Could you check a few things on this model? Use its own coordinates, in mm. Round coordinates to 2 decimals unless told otherwise and drop trailing zeros. Write each loop counter-clockwise with the first axis right and the second up, starting at its lowest first coordinate (ties: lowest second). Pieces come first, ordered by that corner, then holes. Notation, with made-up numbers: (-10.75, 52.25) -> (21.25, 52.25) arc R10 ccw to (21.25, 60.25) -> close; hole circle Ø4 at (69.25, -27). An arc over 180 degrees is marked (long way). Answer in a Markdown table with one row per item. Add a question column.
```python
from build123d import *

# Parameters (mm, degrees)
SKETCH1_R           = 1.5
BOSS_EXTRUDE1_DEPTH = 3
SKETCH4_R           = 1.5
CUT_EXTRUDE4_DEPTH  = 165.076201809


with BuildPart() as part:
    # Sketch1 → Boss-Extrude1 (new body)
    with BuildSketch(Plane(origin=(0, 0, 0), x_dir=(1, 0, 0), z_dir=(0, 1, 0))):
        with BuildLine():
            Line((0, 4), (160, 4))
            ThreePointArc((160, 4), (164, 0), (160, -4))
            Line((160, -4), (0, -4))
            ThreePointArc((0, -4), (-4, 0), (0, 4))
        make_face()
        with Locations(Location((0, 0, 0), (0, 0, 270))):
            Circle(SKETCH1_R, mode=Mode.SUBTRACT)
        with Locations(Location((160, 0, 0), (0, 0, 270))):
            Circle(SKETCH1_R, mode=Mode.SUBTRACT)
        with Locations(Location((120, 0, 0), (0, 0, 270))):
            Circle(SKETCH1_R, mode=Mode.SUBTRACT)
    extrude(amount=BOSS_EXTRUDE1_DEPTH)

    # Sketch4 → Cut-Extrude4 (cut, through all)
    with BuildSketch(Plane(origin=(0, 0, 0), x_dir=(1, 0, 0), z_dir=(0, 1, 0))):
        with Locations(Location((40, 0, 0), (0, 0, 270))):
            Circle(SKETCH4_R)
    extrude(amount=CUT_EXTRUDE4_DEPTH, mode=Mode.SUBTRACT)


solid = part.part
```
(1) I need wall thicknesses on L1, parallel to X at y = 0.65, z = 0; L2, parallel to X at y = 2.3, z = -1.25; L3, parallel to Z at x = 120, y = 2. Which ranges of each line are inside material? Lowest first, please.
(2) Suppose I cut it at A-A, the plane z = 0. Please give me the cut outline in (x, y).
(3) For P1, Ø1, axis at y = 1.5, z = -2.5, coming from the +X side; P2, Ø1.8, axis at x = 160, z = 0, coming from the +Y side, each with a flat end and sliding along its axis, tell me the tip position at first contact or that it passes through.
(4) Suppose I cut it at C-C, the plane y = 1.05. Please give me the cut outline in (x, z).
(5) If we mould it in two halves opening along Z, with no side actions, what happens to faces 1 (the face through (81, 1, 4)), 2 (the face through (164, 1, 0)), 3 (the face through (79, 1, -4)), 4 (the face through (161.487, 1.479, -0.195))? For each: pulls with the +Z half, pulls with the -Z half, needs draft (parallel to the pull), parting line crosses it, or undercut.
(6) Suppose I cut it at B-B, the plane x = 120. Please give me the cut outline in (y, z).
Response:
| question | item | result |
|---|---|---|
| 1 | L1 | -4 to -1.5, 1.5 to 38.5, 41.5 to 118.5, 121.5 to 158.5, 161.5 to 164 |
| 1 | L2 | -3.8 to -0.83, 0.83 to 39.17, 40.83 to 119.17, 120.83 to 159.17, 160.83 to 163.8 |
| 1 | L3 | -4 to -1.5, 1.5 to 4 |
| 2 | outline | (-4, 0) -> (-1.5, 0) -> (-1.5, 3) -> (-4, 3) -> close; (1.5, 0) -> (38.5, 0) -> (38.5, 3) -> (1.5, 3) -> close; (41.5, 0) -> (118.5, 0) -> (118.5, 3) -> (41.5, 3) -> close; (121.5, 0) -> (158.5, 0) -> (158.5, 3) -> (121.5, 3) -> close; (161.5, 0) -> (164, 0) -> (164, 3) -> (161.5, 3) -> close |
| 3 | P1 | x = 163.46 |
| 3 | P2 | through |
| 4 | outline | (0, -4) -> (160, -4) arc R4 ccw to (160, 4) -> (0, 4) arc R4 ccw to start; hole circle Ø3 at (0, 0); hole circle Ø3 at (40, 0); hole circle Ø3 at (120, 0); hole circle Ø3 at (160, 0) |
| 5 | face 1 | pulls with the +Z half |
| 5 | face 2 | parting line crosses it |
| 5 | face 3 | pulls with the -Z half |
| 5 | face 4 | undercut |
| 6 | outline | (0, -4) -> (3, -4) -> (3, -1.5) -> (0, -1.5) -> close; (0, 1.5) -> (3, 1.5) -> (3, 4) -> (0, 4) -> close |
